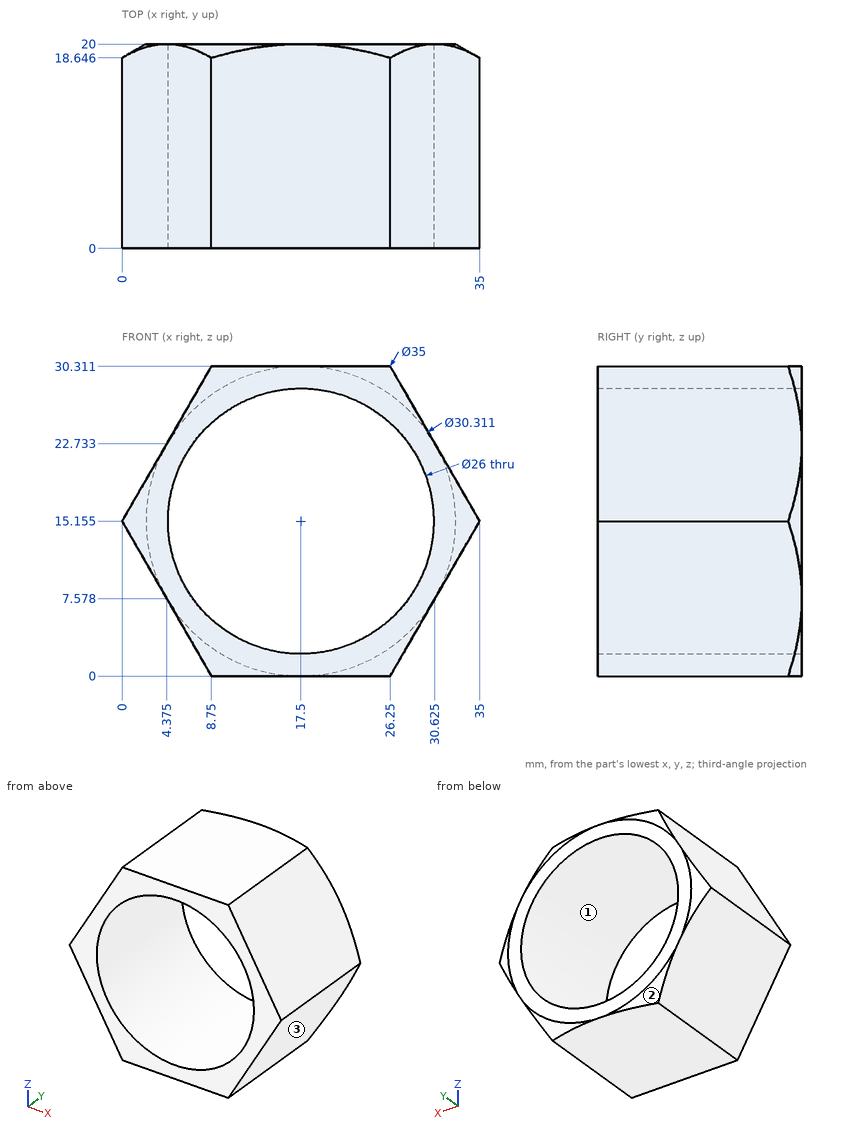
Check sheet for the drawn part. Datum: minimum x, y, z corner. Units: mm. Round coordinates to 2 decimals unless told otherwise and drop trailing zeros. Put each result on its own line as item: value. Start each with the question number.
1. Draft check along X on the marked faces 1, 2 and 3. Enter one of: +X half, -X half, draft (parallel to the pull), parting line (faces both ways), or undercut.
2. Gauge pin test, flat ends, axial feed: pin 1 (1.5 mm diameter, centred on y = 4, z = 26, fed in from +X); pin 2 (1.5 mm diameter, centred on y = 17.5, z = 8, fed in from +X); pin 3 (3 mm diameter, centred on y = 7.5, z = 15, fed in from -X). Record the tip position at first contact, or that the pin passes through.
3. Scan lines: probe 1 along Z at (x, y) = (17.5, 14.25) (1 decimal); probe 2 along X at (y, z) = (6.25, 10.5); probe 3 along X at (y, z) = (1.5, 15). Record each from-to range of solid material in increasing order.
Findings:
1. face 1: undercut
1. face 2: -X half
1. face 3: +X half
2. pin 1: stops at x = 29.17
2. pin 2: stops at x = 31.3
2. pin 3: stops at x = 0
3. probe 1: z = 0 to 2.2, 28.2 to 30.3
3. probe 2: x = 2.69 to 5.36, 29.64 to 32.31
3. probe 3: x = 0.09 to 4.5, 30.5 to 34.91
